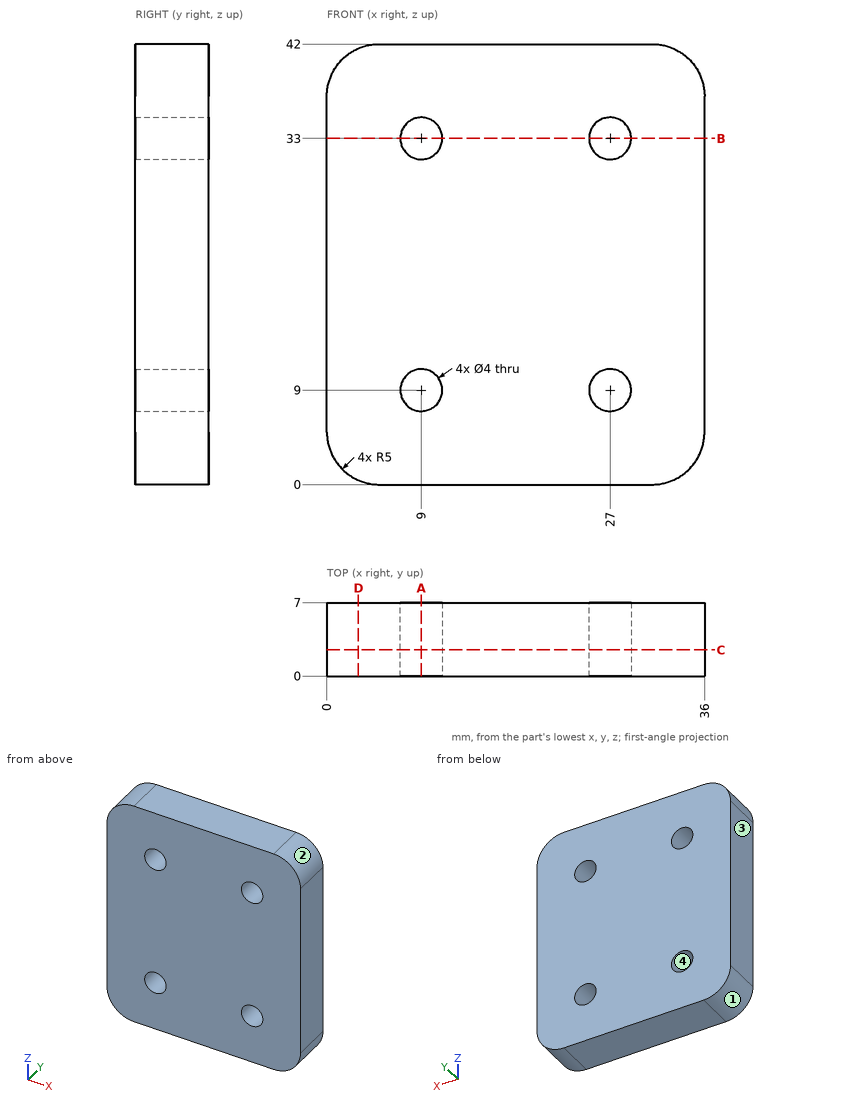
Input: dimensioned drawing with shaded views. Units: mm. Origin: part minimum x, y, z. Give positions to 0.01 mm unless a question says otherwise; leave off trailing zeros. Order: outer loops, then holes, each group sorted by start corner. A loop starts at its lowest first (then second) coordinate and runs counter-clockwise, first axis right, second up.
(1) Section query D-D (x = 3). Return the cut outline in (y, z), plus the area to 3 significant figures.
(2) Pull-direction query (Z, two-part tool) for the marked faces 1, 2, 3 and 4; classes: +Z half, -Z half, draft (parallel to the pull), parting line (faces both ways), or undercut.
(3) Section query A-A (x = 9). Return the cut outline in (y, z).
(4) Material intervals for line 1 along Z through (x, y) = (27, 2); line 2 along X through (y, z) = (3.5, 32); line 3 along Z through (x, y) = (27.5, 6), sorted ascending.
(5) Section query B-B (z = 33). Return the cut outline in (x, y), plus the area to 3 significant figures.
(6) Section query C-C (y = 2.5). Return the cut outline in (x, z), plus the area to 3 significant figures.
Outcome:
1. outline: (0, 0.42) - (7, 0.42) - (7, 41.58) - (0, 41.58) - close
1. area: 288 mm2
2. face 1: -Z half
2. face 2: +Z half
2. face 3: draft
2. face 4: undercut
3. outline: (0, 0) - (7, 0) - (7, 7) - (0, 7) - close; (0, 11) - (7, 11) - (7, 31) - (0, 31) - close; (0, 35) - (7, 35) - (7, 42) - (0, 42) - close
4. line 1: z = 0 to 7, 11 to 31, 35 to 42
4. line 2: x = 0 to 7.27, 10.73 to 25.27, 28.73 to 36
4. line 3: z = 0 to 7.06, 10.94 to 31.06, 34.94 to 42
5. outline: (0, 0) - (7, 0) - (7, 7) - (0, 7) - close; (11, 0) - (25, 0) - (25, 7) - (11, 7) - close; (29, 0) - (36, 0) - (36, 7) - (29, 7) - close
5. area: 196 mm2
6. outline: (0, 5) arc R5 ccw to (5, 0) - (31, 0) arc R5 ccw to (36, 5) - (36, 37) arc R5 ccw to (31, 42) - (5, 42) arc R5 ccw to (0, 37) - close; hole circle Ø4 at (9, 9); hole circle Ø4 at (9, 33); hole circle Ø4 at (27, 9); hole circle Ø4 at (27, 33)
6. area: 1,440 mm2
